Source: CAD feature listing. Evaluate the final solid. Frame: model axes, mm. Face numbers are marked on the shaded views. A direction names the side the tool comes from. Give positions to 0.01 mm unless a question says otherwise; leave off trailing zeros. Loops run counter-clockwise (first coordinate to the right, second up) from the corner with the lowest first, then second, coordinate; pieces in that order, holes last. Notation, with made-up numbers: (59.5, 81.5) - (107.5, 81.5) arc R22 cw to (107.5, 113.5) - close; hole circle Ø5 at (86.5, 75.5). An arc over 180 degrees is marked (long way). Put each result on its own line as item: value.
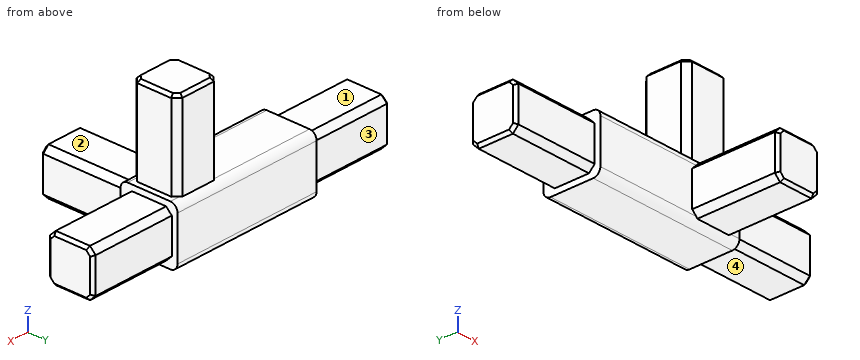
```python
from build123d import *

# Parameters (mm, degrees)
F0_W          = 16
F0_H          = 16
F1_DEPTH      = 50
F0_W_2        = 20
F0_H_2        = 20
F2_DEPTH      = 20
F3_W          = 16
F3_H          = 16
F4_DEPTH      = 40
F5_W          = 16
F5_H          = 16
F6_DEPTH      = 73
F7_W          = 16
F7_H          = 16
F8_DEPTH      = 40
F9_DEPTH      = 33
F10_T1_DEPTH  = 65.5
F10_T6_DEPTH  = 65.5
F10_T11_DEPTH = 65.5
F10_T17_DEPTH = 65.5
F10_T22_DEPTH = 65.5
F10_T27_DEPTH = 65.5
F10_T32_DEPTH = 65.5
F10_T37_DEPTH = 65.5
F10_T42_DEPTH = 65.5
F10_T47_DEPTH = 65.5
F11_SIZE      = 2
F12_SIZE      = 1


# Not quite as in the source:
# - a fillet or chamfer that OpenCascade refuses, or shapes differently, is made with other operations: its cross-section is extruded or revolved along the edge and cut away or added


with BuildPart() as f1:
    # F0 (on Front) → F1 (new body)
    with BuildSketch(Plane.XZ):
        Rectangle(F0_W, F0_H)
    extrude(amount=F1_DEPTH)

    # F0 (on Front) → F2 (join)
    with BuildSketch(Plane.XZ):
        Rectangle(F0_W_2, F0_H_2)
        Rectangle(F0_W, F0_H, mode=Mode.SUBTRACT)
    extrude(amount=F2_DEPTH)

    # F3 (on Right) → F4 (join)
    with BuildSketch(Plane.YZ):
        with Locations((-10, 0)):
            Rectangle(F3_W, F3_H)
    extrude(amount=F4_DEPTH)

    # F5 (on Right) → F6 (join)
    with BuildSketch(Plane.YZ):
        with Locations((-10, 0)):
            Rectangle(F5_W, F5_H)
    extrude(amount=-F6_DEPTH)

    # F7 (on Top) → F8 (join)
    with BuildSketch(Plane.XY):
        with Locations((0, -10)):
            Rectangle(F7_W, F7_H)
    extrude(amount=F8_DEPTH)

    # F9 (add): a face of the model
    f9_faces = [f1.faces().sort_by_distance(p)[0] for p in [
        (-10, -10, 9.7171572875),
    ]]
    extrude(f9_faces, amount=F9_DEPTH)

    # F10: fillet of radius 2.5 on 4 edges, made by hand

    # F10_s2 → F10_t1 (cut)
    with BuildSketch(Plane.YZ.offset(-49.25)):
        with BuildLine():
            ThreePointArc((-2.5, -10), (-0.732233047, -9.267766953), (0, -7.5))
            Line((0, -7.5), (0, -10))
            Line((0, -10), (-2.5, -10))
        make_face()
    extrude(amount=F10_T1_DEPTH, mode=Mode.SUBTRACT)


with BuildPart() as f10_tool4:
    # F10_s5 → F10_t6 (new body)
    with BuildSketch(Plane.YZ.offset(16.25)):
        with BuildLine():
            ThreePointArc((-20, 7.5), (-19.267766953, 9.267766953), (-17.5, 10))
            Line((-17.5, 10), (-20, 10))
            Line((-20, 10), (-20, 7.5))
        make_face()
    extrude(amount=-F10_T6_DEPTH)

    split(bisect_by=Plane.YZ.offset(8), keep=Keep.TOP)


with BuildPart() as f1_1:
    add(f1.part)

    # F10_t3: cut F10_tool4
    add(f10_tool4.part, mode=Mode.SUBTRACT)


with BuildPart() as f10_tool9:
    # F10_s10 → F10_t11 (new body)
    with BuildSketch(Plane.YZ.offset(16.25)):
        with BuildLine():
            ThreePointArc((-20, 7.5), (-19.267766953, 9.267766953), (-17.5, 10))
            Line((-17.5, 10), (-20, 10))
            Line((-20, 10), (-20, 7.5))
        make_face()
    extrude(amount=-F10_T11_DEPTH)

    split(bisect_by=Plane.XY.offset(8), keep=Keep.TOP)

    split(bisect_by=Plane.XZ.offset(18), keep=Keep.TOP)


with BuildPart() as f1_2:
    add(f1_1.part)

    # F10_t8: cut F10_tool9
    add(f10_tool9.part, mode=Mode.SUBTRACT)


with BuildPart() as f10_tool15:
    # F10_s16 → F10_t17 (new body)
    with BuildSketch(Plane.YZ.offset(16.25)):
        with BuildLine():
            ThreePointArc((-20, 7.5), (-19.267766953, 9.267766953), (-17.5, 10))
            Line((-17.5, 10), (-20, 10))
            Line((-20, 10), (-20, 7.5))
        make_face()
    extrude(amount=-F10_T17_DEPTH)

    split(bisect_by=Plane.YZ.offset(-8), keep=Keep.BOTTOM)


with BuildPart() as f1_3:
    add(f1_2.part)

    # F10_t14: cut F10_tool15
    add(f10_tool15.part, mode=Mode.SUBTRACT)


with BuildPart() as f10_tool20:
    # F10_s21 → F10_t22 (new body)
    with BuildSketch(Plane.YZ.offset(-49.25)):
        with BuildLine():
            ThreePointArc((-20, -7.5), (-19.267766953, -9.267766953), (-17.5, -10))
            Line((-17.5, -10), (-20, -10))
            Line((-20, -10), (-20, -7.5))
        make_face()
    extrude(amount=F10_T22_DEPTH)

    split(bisect_by=Plane.YZ.offset(-8), keep=Keep.BOTTOM)


with BuildPart() as f1_4:
    add(f1_3.part)

    # F10_t19: cut F10_tool20
    add(f10_tool20.part, mode=Mode.SUBTRACT)


with BuildPart() as f10_tool25:
    # F10_s26 → F10_t27 (new body)
    with BuildSketch(Plane.YZ.offset(-49.25)):
        with BuildLine():
            ThreePointArc((-20, -7.5), (-19.267766953, -9.267766953), (-17.5, -10))
            Line((-17.5, -10), (-20, -10))
            Line((-20, -10), (-20, -7.5))
        make_face()
    extrude(amount=F10_T27_DEPTH)

    split(bisect_by=Plane.XY.offset(-8), keep=Keep.BOTTOM)


with BuildPart() as f1_5:
    add(f1_4.part)

    # F10_t24: cut F10_tool25
    add(f10_tool25.part, mode=Mode.SUBTRACT)


with BuildPart() as f10_tool30:
    # F10_s31 → F10_t32 (new body)
    with BuildSketch(Plane.YZ.offset(-49.25)):
        with BuildLine():
            ThreePointArc((-20, -7.5), (-19.267766953, -9.267766953), (-17.5, -10))
            Line((-17.5, -10), (-20, -10))
            Line((-20, -10), (-20, -7.5))
        make_face()
    extrude(amount=F10_T32_DEPTH)

    split(bisect_by=Plane.YZ.offset(8), keep=Keep.TOP)


with BuildPart() as f1_6:
    add(f1_5.part)

    # F10_t29: cut F10_tool30
    add(f10_tool30.part, mode=Mode.SUBTRACT)


with BuildPart() as f10_tool35:
    # F10_s36 → F10_t37 (new body)
    with BuildSketch(Plane.YZ.offset(16.25)):
        with BuildLine():
            ThreePointArc((0, 7.5), (-0.732233047, 9.267766953), (-2.5, 10))
            Line((-2.5, 10), (0, 10))
            Line((0, 10), (0, 7.5))
        make_face()
    extrude(amount=-F10_T37_DEPTH)

    split(bisect_by=Plane.XZ.offset(2), keep=Keep.BOTTOM)


with BuildPart() as f1_7:
    add(f1_6.part)

    # F10_t34: cut F10_tool35
    add(f10_tool35.part, mode=Mode.SUBTRACT)


with BuildPart() as f10_tool40:
    # F10_s41 → F10_t42 (new body)
    with BuildSketch(Plane.YZ.offset(16.25)):
        with BuildLine():
            ThreePointArc((0, 7.5), (-0.732233047, 9.267766953), (-2.5, 10))
            Line((-2.5, 10), (0, 10))
            Line((0, 10), (0, 7.5))
        make_face()
    extrude(amount=-F10_T42_DEPTH)

    split(bisect_by=Plane.YZ.offset(8), keep=Keep.TOP)


with BuildPart() as f1_8:
    add(f1_7.part)

    # F10_t39: cut F10_tool40
    add(f10_tool40.part, mode=Mode.SUBTRACT)


with BuildPart() as f10_tool45:
    # F10_s46 → F10_t47 (new body)
    with BuildSketch(Plane.YZ.offset(16.25)):
        with BuildLine():
            ThreePointArc((0, 7.5), (-0.732233047, 9.267766953), (-2.5, 10))
            Line((-2.5, 10), (0, 10))
            Line((0, 10), (0, 7.5))
        make_face()
    extrude(amount=-F10_T47_DEPTH)

    split(bisect_by=Plane.YZ.offset(-8), keep=Keep.BOTTOM)


with BuildPart() as f1_9:
    add(f1_8.part)

    # F10_t44: cut F10_tool45
    add(f10_tool45.part, mode=Mode.SUBTRACT)

    # F11
    f11_edges = [f1_9.edges().sort_by_distance(p)[0] for p in [
        (-58, -18, 8),
        (-58, -18, -8),
        (-58, -2, 8),
        (-58, -2, -8),
        (-8, -34.974745, 8),
        (-8, -34.974745, -8),
        (8, -34.974745, 8),
        (8, -34.974745, -8),
        (25, -18, -8),
        (25, -18, 8),
        (8, -18, 24.974745),
        (-8, -18, 24.974745),
        (25, -2, -8),
        (25, -2, 8),
        (8, -2, 24.974745),
        (-8, -2, 24.974745),
    ]]
    chamfer(f11_edges, length=F11_SIZE)

    # F12
    f12_edges = [f1_9.edges().sort_by_distance(p)[0] for p in [
        (-73, -10, 8),
        (-73, -10, -8),
        (-73, -17, -7),
        (-73, -3, -7),
        (-73, -18, 0),
        (-73, -2, 0),
        (-73, -17, 7),
        (-73, -3, 7),
        (-8, -50, 0),
        (-7, -50, 7),
        (-7, -50, -7),
        (0, -50, 8),
        (0, -50, -8),
        (7, -50, 7),
        (7, -50, -7),
        (8, -50, 0),
        (-8, -10, 40),
        (-7, -3, 40),
        (-7, -17, 40),
        (0, -2, 40),
        (0, -18, 40),
        (7, -3, 40),
        (7, -17, 40),
        (8, -10, 40),
        (40, -10, -8),
        (40, -17, -7),
        (40, -3, -7),
        (40, -18, 0),
        (40, -2, 0),
        (40, -17, 7),
        (40, -3, 7),
        (40, -10, 8),
    ]]
    chamfer(f12_edges, length=F12_SIZE)


solid = f1_9.part
```
1) Access query for the marked faces 1, 2, 3 and 4. Directions: +Z, -Z, +X, -X, +Y, -Y. A direction counts if a zero-diameter tool reaches every point of the face in a straight line with its end or side. Return the directions, or none.
Check result:
face 1: +Z, -X, +Y, -Y
face 2: +Z, +X, -X, -Y
face 3: +Z, -Z, -X, +Y
face 4: -Z, +X, +Y, -Y
2) Pin query (flat end, axial travel): P1, Ø1, axis at x = 24.5, y = -16, coming from the +Z side; P2, Ø5, axis at x = -43.5, y = -21.5, coming from the -Z side; P3, Ø6, axis at x = 23.5, y = -9.5, coming from the -Z side. Return the tip coordinate at first contact, or that it passes through.
Check result:
P1: z = 8
P2: z = -9.46
P3: z = -8
3) Section query C-C, the plane z = -0.5. Output: boundary loops of the cut face in (x, y).
Check result:
outline: (-73, -17) - (-72, -18) - (-43, -18) - (-43, -20) - (-8, -20) - (-8, -49) - (-7, -50) - (7, -50) - (8, -49) - (8, -20) - (10, -20) - (10, -18) - (39, -18) - (40, -17) - (40, -3) - (39, -2) - (10, -2) - (10, 0) - (-43, 0) - (-43, -2) - (-72, -2) - (-73, -3) - close
4) Material intervals for line 1 along Y through (x, z) = (-38.5, -7); line 2 along X through (y, z) = (-4, 27.5); line 3 along Y through (x, z) = (-53.5, -0.5), sorted ascending. Write a range as [from, to].
Check result:
line 1: [-20, 0]
line 2: [-8, 8]
line 3: [-18, -2]
5) Section query B-B, the plane x = 4. Output: boundary loops of the cut face in (y, z).
Check result:
outline: (-50, -7) - (-49, -8) - (-19.95, -8) arc R2.5 ccw to (-17.5, -10) - (-2.5, -10) arc R2.5 ccw to (0, -7.5) - (0, 7.5) arc R2.5 ccw to (-2, 9.95) - (-2, 39) - (-3, 40) - (-17, 40) - (-18, 39) - (-18, 9.95) arc R2.5 ccw to (-19.95, 8) - (-49, 8) - (-50, 7) - close
6) Section query D-D, the plane y = -6. Output: boundary loops of the cut face in (x, z), plus the area to 3 significant figures.
Check result:
outline: (-73, -7) - (-72, -8) - (-43, -8) - (-43, -10) - (10, -10) - (10, -8) - (39, -8) - (40, -7) - (40, 7) - (39, 8) - (10, 8) - (10, 10) - (8, 10) - (8, 39) - (7, 40) - (-7, 40) - (-8, 39) - (-8, 10) - (-43, 10) - (-43, 8) - (-72, 8) - (-73, 7) - close
area: 2,500 mm²
7) Section query A-A, the plane y = -22. Output: boundary loops of the cut face in (x, z).
Check result:
outline: (-8, -6) - (-6, -8) - (6, -8) - (8, -6) - (8, 6) - (6, 8) - (-6, 8) - (-8, 6) - close
